from build123d import *

# Parameters (mm, degrees)
F0_W     = 62.8
F0_H     = 54
F0_W_2   = 12.8
F0_H_2   = 14
F0_W_3   = 11.6
F0_H_3   = 12.8
F0_W_4   = 10.6
F0_H_4   = 11.8
F1_DEPTH = 0.5
F2_DEPTH = 1


with BuildPart() as f1:
    # F0 (on Top) → F1 (new body)
    with BuildSketch(Plane.XY):
        with Locations((15, 10)):
            Rectangle(F0_W, F0_H)
        Rectangle(F0_W_2, F0_H_2, mode=Mode.SUBTRACT)
        Rectangle(F0_W_2, F0_H_2)
        Rectangle(F0_W_3, F0_H_3, mode=Mode.SUBTRACT)
        Rectangle(F0_W_3, F0_H_3)
        Rectangle(F0_W_4, F0_H_4, mode=Mode.SUBTRACT)
    extrude(amount=F1_DEPTH)

    # F0 (on Top) → F2 (join)
    with BuildSketch(Plane.XY):
        Rectangle(F0_W_3, F0_H_3)
        Rectangle(F0_W_4, F0_H_4, mode=Mode.SUBTRACT)
    extrude(amount=F2_DEPTH)


solid = f1.part
The model under review builds one solid part; all positions refer to its coordinate system, in mm. Round coordinates to 2 decimals unless told otherwise and drop trailing zeros. Write each loop counter-clockwise with the first axis right and the second up, starting at its lowest first coordinate (ties: lowest second). Pieces come first, ordered by that corner, then holes. Notation, with made-up numbers: (-14.75, 25) -> (-3.75, 25) arc R24 cw to (-3.75, 52) -> close; hole circle Ø7 at (40.5, -4.5). An arc over 180 degrees is marked (long way). Answer as a JSON object with one key per item and string values.
1. We need section A-A on y = -2. State the section outline as (x, z) points.
Results found:
{"outline": "(-16.4, 0) -> (-5.3, 0) -> (-5.3, 1) -> (-5.8, 1) -> (-5.8, 0.5) -> (-16.4, 0.5) -> close; (5.3, 0) -> (46.4, 0) -> (46.4, 0.5) -> (5.8, 0.5) -> (5.8, 1) -> (5.3, 1) -> close"}
2. We need section D-D on x = 13. State the section outline as (y, z) points, and give its area (3 significant figures).
Results found:
{"outline": "(-17, 0) -> (37, 0) -> (37, 0.5) -> (-17, 0.5) -> close", "area": "27.0 mm^2"}
3. We need section B-B on z = 0.75. State the section outline as (x, y) points.
Results found:
{"outline": "(-5.8, -6.4) -> (5.8, -6.4) -> (5.8, 6.4) -> (-5.8, 6.4) -> close; hole (-5.3, -5.9) -> (5.3, -5.9) -> (5.3, 5.9) -> (-5.3, 5.9) -> close"}
4. We need section C-C on x = -2.5. State the section outline as (y, z) points, and give its area (3 significant figures).
Results found:
{"outline": "(-17, 0) -> (-5.9, 0) -> (-5.9, 1) -> (-6.4, 1) -> (-6.4, 0.5) -> (-17, 0.5) -> close; (5.9, 0) -> (37, 0) -> (37, 0.5) -> (6.4, 0.5) -> (6.4, 1) -> (5.9, 1) -> close", "area": "21.6 mm^2"}
5. Clearance check with flat-ended pins moving along their axes: pin 1 (8 mm diameter, centred on x = 26.5, y = 15.5, fed in from +Z); pin 2 (3 mm diameter, centred on x = -1.5, y = 13, fed in from -Z); pin 3 (0.6 mm diameter, centred on x = 0.5, z = 1, fed in from -Y). State where each tip first meets the part, or that it passes through.
Results found:
{"pin 1": "stops at z = 0.5", "pin 2": "stops at z = 0", "pin 3": "stops at y = -6.4"}
6. To check wall thickness, follow line 1 along Y through (x, z) = (0, 0.1); line 2 along X through (y, z) = (-5.5, 0.95); line 3 along Z through (x, y) = (42.5, 18.5). State the ranges of each line that lie inside material, in increasing order.
Results found:
{"line 1": "y = -17 to -5.9, 5.9 to 37", "line 2": "x = -5.8 to -5.3, 5.3 to 5.8", "line 3": "z = 0 to 0.5"}
